from build123d import *


with BuildPart() as f1:
    # F0 (on Right) → F1 (revolve)
    with BuildSketch(Plane.YZ):
        with BuildLine():
            ThreePointArc((0, 2), (3.939137, 1.499026), (7.616186, 0))
            Line((7.616186, 0), (9.116186, 0))
            Line((9.116186, 0), (9.116186, 2.46))
            Line((9.116186, 2.46), (5.95, 2.46))
            Line((5.95, 2.46), (5.95, 3.46))
            Line((5.95, 3.46), (3.8, 3.46))
            Line((3.8, 3.46), (3.8, 6.46))
            Line((3.8, 6.46), (0, 6.46))
            Line((0, 6.46), (0, 2))
        make_face()
    revolve(axis=Axis((0, 0, 3.23), (0, 0, -1)))


solid = f1.part
Design review of the part built by this model. Coordinates are the model's own, in mm. A direction names the side the tool comes from. Give positions to 0.01 mm unless a question says otherwise; leave off trailing zeros. Loops run counter-clockwise (first coordinate to the right, second up) from the corner with the lowest first, then second, coordinate; pieces in that order, holes last. Notation, with made-up numbers: M 18.25,-12 L 56.25,-12 A16 ccw 56.25,18 Z; hole C 80,85 d2. An arc over 180 degrees is marked long. Answer as a JSON object with one key per item and string values.
Item 1: We need section C-C (z = 3). State the section outline as (x, y) points.
Output values:
{"outline": "C 0,0 d11.9"}
Item 2: We need section A-A (z = 5). State the section outline as (x, y) points, and give its area (3 significant figures).
Output values:
{"outline": "C 0,0 d7.6", "area": "45.4 mm2"}
Item 3: We need section B-B (x = 8.25). State the section outline as (y, z) points.
Output values:
{"outline": "M -3.88,0 L 3.88,0 L 3.88,2.46 L -3.88,2.46 Z"}
Item 4: Machinability: for faces 1 (the face through (-6, 2, 2.46)), 2 (the face through (0, 0, 6.46)), which of the approach directions +Z, -Z, +X, -X, +Y, -Y give a long, thin tool a straight path to every point of the face, cutting with its end or side? Answer none if there is none.
Output values:
{"face 1": "+Z", "face 2": "+Z, +X, -X, +Y, -Y"}
Item 5: For P1, Ø1, axis at x = 0, z = 5.5, coming from the +Y side; P2, Ø6, axis at x = 7, y = 5.5, coming from the +Z side; P3, Ø1.5, axis at y = -2.5, z = 1.5, coming from the +X side, all flat-tipped, find the tip position at first contact; note any pin that passes through.
Output values:
{"P1": "stops at y = 3.8", "P2": "stops at z = 3.46", "P3": "stops at x = 8.95"}
Item 6: Wall thickness on line 1 along Z through (x, y) = (-7, 3.25); line 2 along X through (y, z) = (-3.5, 3); line 3 along X through (y, z) = (-1.5, 3.25): over which ranges is each line inside the solid? List them lowest first.
Output values:
{"line 1": "z = 0 to 2.46", "line 2": "x = -4.81 to 4.81", "line 3": "x = -5.76 to 5.76"}
